Input: part model. Units: mm. Frame: model coordinates. Face numbers are marked on the shaded views. Round coordinates to 2 decimals unless told otherwise and drop trailing zeros. Order: outer loops, then holes, each group sorted by start corner. A loop starts at its lowest first (then second) coordinate and runs counter-clockwise, first axis right, second up. Notation, with made-up numbers: (64, 48.5) - (81, 48.5) arc R22 cw to (81, 87.5) - close; hole circle Ø1 at (24.25, 87). An arc over 180 degrees is marked (long way). One line per item, written item: value. Start each with the question number.
from build123d import *

# Parameters (mm, degrees)
F0_R          = 1.5
F0_R_2        = 4.25
F1_DEPTH      = 1.25
F2_R          = 15
F2_R_2        = 1.5
F2_R_3        = 4.25
F3_DEPTH      = 2
F5_DEPTH      = 2
F5_DEPTH_BACK = 0.75
F6_R          = 1


with BuildPart() as f1:
    # F0 (on Front) → F1 (new body, symmetric)
    with BuildSketch(Plane.XZ):
        with BuildLine():
            Line((4, 17.75), (0, 17.75))
            Line((0, 17.75), (-4, 17.75))
            add(Edge.make_bspline(
                [(-4, 17.75), (-10.6686704129, 17.75), (-19.5, 9.0568709765), (-19.5, 4.25)],
                knots=[0, 0, 0, 0, 20.5548047911, 20.5548047911, 20.5548047911, 20.5548047911], degree=3))
            Line((-19.5, 4.25), (-19.5, -17.75))
            Line((-19.5, -17.75), (19.5, -17.75))
            Line((19.5, -17.75), (19.5, 4.25))
            add(Edge.make_bspline(
                [(4, 17.75), (10.6686704129, 17.75), (19.5, 9.0568709765), (19.5, 4.25)],
                knots=[0, 0, 0, 0, 20.5548047911, 20.5548047911, 20.5548047911, 20.5548047911], degree=3))
        make_face()
        with Locations((-6.6568542495, -5.4068542495)):
            Circle(F0_R, mode=Mode.SUBTRACT)
        with Locations((4.6568542495, -5.4068542495)):
            Circle(F0_R, mode=Mode.SUBTRACT)
        with Locations((-1, 0.25)):
            Circle(F0_R_2, mode=Mode.SUBTRACT)
        with Locations((-6.6568542495, 5.9068542495)):
            Circle(F0_R, mode=Mode.SUBTRACT)
        with Locations((4.6568542495, 5.9068542495)):
            Circle(F0_R, mode=Mode.SUBTRACT)
    extrude(amount=F1_DEPTH, both=True)

    # F2 (on Front) → F3 (join)
    with BuildSketch(Plane.XZ):
        with Locations((-1, 0.25)):
            Circle(F2_R)
        with Locations((-6.6568542495, -5.4068542495)):
            Circle(F2_R_2, mode=Mode.SUBTRACT)
        with Locations((4.6568542495, -5.4068542495)):
            Circle(F2_R_2, mode=Mode.SUBTRACT)
        with Locations((-6.6568542495, 5.9068542495)):
            Circle(F2_R_2, mode=Mode.SUBTRACT)
        with Locations((-1, 0.25)):
            Circle(F2_R_3, mode=Mode.SUBTRACT)
        with Locations((4.6568542495, 5.9068542495)):
            Circle(F2_R_2, mode=Mode.SUBTRACT)
    extrude(amount=F3_DEPTH)

    # F4 (on face) → F5 (join, two sides)
    with BuildSketch(Plane.XZ.offset(2)) as f5_sk:
        Polygon((19.5, -1.75), (19.5, -1.25), (19.5, -0.75), (11.7, -0.75), (11.7, -1.25), (11.7, -1.75), align=None)
    extrude(amount=F5_DEPTH)
    extrude(f5_sk.sketch, amount=-F5_DEPTH_BACK)

    # F6
    f6_edges = [f1.edges().sort_by_distance(p)[0] for p in [
        (19.5, 0, -17.75),
        (-19.5, 0, -17.75),
    ]]
    fillet(f6_edges, radius=F6_R)


solid = f1.part
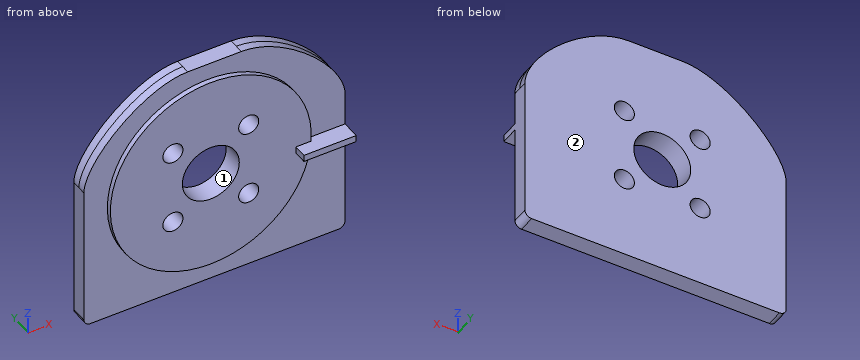
1. Line query: line 1 (X direction, y = -1, z = -5.5); line 2 (Z direction, x = 6, y = -1.95); line 3 (X direction, y = 0.55, z = -4.5). Output: solid intervals per line, ascending. Write a range as from..to.
2. Section D-D (y = -3.5). Return the cut outline in (x, z), then the cut area to 3 significant figures.
3. Section C-C (z = -7.5). Return the cut outline in (x, y), then the cut area to 3 significant figures.
4. Pull-direction query (X, two-part tool) for the marked faces 1 and 2; classes: released by +X, released by -X, zero draft, split by the parting line, or undercut.
5. Section B-B (z = 0.25). Return the cut outline in (x, y), then the cut area to 3 significant figures.
6. Pin query (flat end, axial travel): pin 1 (10.5 mm diameter, centred on x = 0.5, z = 1.5, fed in from -Y); pin 2 (3 mm diameter, centred on x = 17.5, y = -2.5, fed in from +Z); pin 3 (0.5 mm diameter, centred on y = -3, z = -1.5, fed in from -X); pin 4 (7 mm diameter, centred on x = -1, z = 0.25, fed in from +Y). Return the tip coordinate at first contact, or that it passes through.
7. Section A-A (x = -1). Return the cut outline in (y, z).
Solved:
1. line 1: x = -19.5..-8.15, -5.16..3.16, 6.15..19.5
1. line 2: z = -13.02..-6.07, -4.74..5.24, 6.57..13.52
1. line 3: x = -19.5..-7.85, -5.46..3.46, 5.85..19.5
2. outline: (11.7, -1.75) - (19.5, -1.75) - (19.5, -0.75) - (11.7, -0.75) - close
2. area: 7.80 mm²
3. outline: (-19.5, -1.25) - (-13.84, -1.25) - (-13.84, -2) - (11.84, -2) - (11.84, -1.25) - (19.5, -1.25) - (19.5, 1.25) - (-19.5, 1.25) - close
3. area: 117 mm²
4. face 1: undercut
4. face 2: zero draft
5. outline: (-19.5, -1.25) - (-16, -1.25) - (-16, -2) - (-5.25, -2) - (-5.25, 1.25) - (-19.5, 1.25) - close; (3.25, -2) - (14, -2) - (14, -1.25) - (19.5, -1.25) - (19.5, 1.25) - (3.25, 1.25) - close
5. area: 92.4 mm²
6. pin 1: stops at y = -2
6. pin 2: stops at z = 10.25
6. pin 3: stops at x = 11.7
6. pin 4: passes through
7. outline: (-2, -14.75) - (-1.25, -14.75) - (-1.25, -17.75) - (1.25, -17.75) - (1.25, -4) - (-2, -4) - close; (-2, 4.5) - (1.25, 4.5) - (1.25, 17.75) - (-1.25, 17.75) - (-1.25, 15.25) - (-2, 15.25) - close
